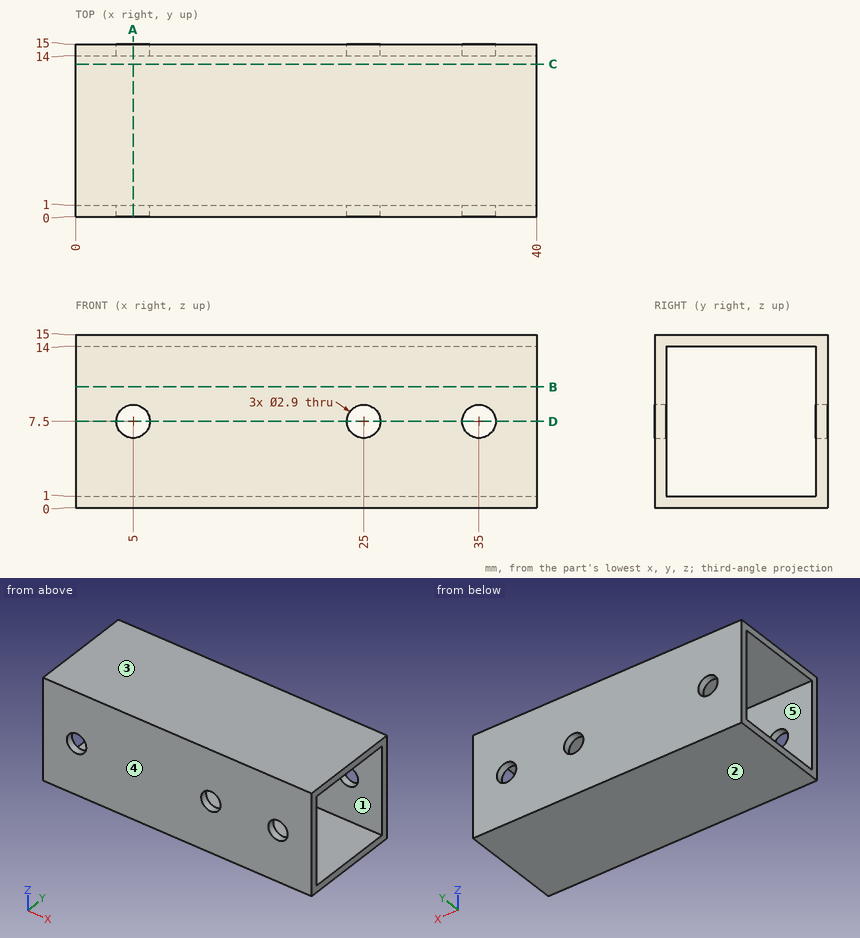
Here's the drawing with two shaded views (mm, measured from the low corner). I have some questions. A direction names the side the tool comes from. Round coordinates to 2 decimals unless told otherwise and drop trailing zeros. Write each loop counter-clockwise with the first axis right and the second up, starting at its lowest first coordinate (ties: lowest second). Pieces come first, ordered by that corner, then holes. Notation, with made-up numbers: M 79,48.5 L 114,48.5 A9 cw 114,52.5 Z; hole C -23,16.25 d5. An arc over 180 degrees is marked long. Answer in a Markdown table with one row per item. Add a question column.
Q1. Imagine slicing it at A-A (x = 5). Please give me the cut outline in (y, z).
Q2. On a 3-axis mill with a long thin cutter (end or side, diameter ignored), from which of +Z, -Z, +X, -X, +Y, -Y can I reach the whole of each face in a straight line? I mean the marked faces 1 and 2. Say none if no direction works.
Q3. Will this pin go through, and if not, where does the flat tip stop? pin 1 Ø6 at (x, z) = (8, 5) entering from -Y.
Q4. If we mould it in two halves opening along Z, with no side actions, what happens to the marked faces 3, 4 and 5? For each: +Z half, -Z half, draft (parallel to the pull), parting line (faces both ways), or undercut.
Q5. If I drill on line 1 (X direction, y = 0.4, z = 7.5); line 2 (Y direction, x = 32.5, z = 4), over which ranges is the centre line in solid material (lowest first)? Write a range as from..to.
Q6. Imagine slicing it at B-B (z = 10.5). Please give me the cut outline in (x, y), then the cut area to 3 significant figures.
Q7. Imagine slicing it at D-D (z = 7.5). Give the number of separate pieces and of enclosed holes in the cut face, then the cut area to 3 significant figures.
Values:
| question | item | result |
|---|---|---|
| 1 | outline | M 0,0 L 15,0 L 15,6.05 L 14,6.05 L 14,1 L 1,1 L 1,6.05 L 0,6.05 Z; M 0,8.95 L 1,8.95 L 1,14 L 14,14 L 14,8.95 L 15,8.95 L 15,15 L 0,15 Z |
| 2 | face 1 | +X, -X |
| 2 | face 2 | -Z, +X, -X, +Y, -Y |
| 3 | pin 1 | y = 0 |
| 4 | face 3 | +Z half |
| 4 | face 4 | draft |
| 4 | face 5 | undercut |
| 5 | line 1 | 0..3.55, 6.45..23.55, 26.45..33.55, 36.45..40 |
| 5 | line 2 | 0..1, 14..15 |
| 6 | outline | M 0,0 L 40,0 L 40,1 L 0,1 Z; M 0,14 L 40,14 L 40,15 L 0,15 Z |
| 6 | area | 80.0 mm^2 |
| 7 | separate pieces | 8 |
| 7 | enclosed holes | 0 |
| 7 | area | 62.6 mm^2 |
